```python
from build123d import *

# Parameters (mm, degrees)
SKETCH1_R           = 3.175
BOSS_EXTRUDE1_DEPTH = 3.175
SKETCH2_W           = 63.5
SKETCH2_H           = 25.4
SKETCH2_R           = 3.175
BOSS_EXTRUDE2_DEPTH = 3.175
FILLET1_R           = 2.54


with BuildPart() as part:
    # Sketch1 → Boss-Extrude1 (new body)
    with BuildSketch(Plane.XY):
        with BuildLine():
            Line((-41.275, 55.28710968), (-41.275, -22.225))
            Line((-41.275, -22.225), (22.225, -22.225))
            Line((22.225, -22.225), (22.225, -6.35))
            Line((22.225, -6.35), (-26.194658329, 42.069658329))
            ThreePointArc((-26.194658329, 42.069658329), (-32.769591892, 42.42721549), (-29.935488317, 48.370737627))
            ThreePointArc((-29.935488317, 48.370737627), (-28.368460583, 49.237906002), (-27.763159017, 50.923482141))
            ThreePointArc((-27.763159017, 50.923482141), (-32.032478959, 57.847259125), (-40.154061033, 57.393733943))
            ThreePointArc((-40.154061033, 57.393733943), (-40.977321902, 56.480253631), (-41.275, 55.28710968))
        make_face()
        Circle(SKETCH1_R, mode=Mode.SUBTRACT)
        with Locations((-31.75, 0)):
            Circle(SKETCH1_R, mode=Mode.SUBTRACT)
        with Locations((-31.75, 31.75)):
            Circle(SKETCH1_R, mode=Mode.SUBTRACT)
    extrude(amount=BOSS_EXTRUDE1_DEPTH)

    # Sketch2 → Boss-Extrude2 (add)
    with BuildSketch(Plane(origin=(0, -22.225, 0), x_dir=(1, 0, 0), z_dir=(0, 1, 0))):
        with Locations((-9.525, -15.875)):
            Rectangle(SKETCH2_W, SKETCH2_H)
        with Locations((-9.525, -15.875)):
            Circle(SKETCH2_R, mode=Mode.SUBTRACT)
        with Locations((-31.75, -19.05)):
            Circle(SKETCH2_R, mode=Mode.SUBTRACT)
        with Locations((12.7, -19.05)):
            Circle(SKETCH2_R, mode=Mode.SUBTRACT)
    extrude(amount=BOSS_EXTRUDE2_DEPTH)

    # Fillet1
    fillet1_edges = [part.edges().sort_by_distance(p)[0] for p in [
        (-9.525, -22.225, 0),
    ]]
    fillet(fillet1_edges, radius=FILLET1_R)


solid = part.part
```
The listing builds one solid part. Answer for the finished solid, in the listing's coordinates (mm). A direction names the side the tool comes from. Coordinates: 2 decimals unless noted, no trailing zeros. Loops run counter-clockwise (first coordinate to the right, second up) from the corner with the lowest first, then second, coordinate; pieces in that order, holes last. Notation, with made-up numbers: (-5.5, 1) -> (18.5, 1) arc R21 cw to (18.5, 5) -> close; hole circle Ø9 at (74, 36.5). An arc over 180 degrees is marked (long way). Return JSON: item names as keys, results as strings. Group by question number.
(1) A cutting plane is placed at B-B on x = 12.7. Write down the section's boundary in (y, z) (3 decimals).
(2) Find the intervals of material crossed by probe 1 along Y at (x, z) = (-31.75, 2.2) (3 decimals); probe 2 along Y at (x, z) = (-3, 10.75) (3 decimals); probe 3 along Z at (x, y) = (-15, 0) (3 decimals), in increasing order. Write a range as from..to.
(3) A cutting plane is placed at A-A on y = 0. Write down the section's boundary in (x, z) (3 decimals), and give its area (3 significant figures).
(4) A cutting plane is placed at C-C on z = 17.25. Write down the section's boundary in (x, y) (3 decimals).
(5) A cutting plane is placed at D-D on x = -31.75. Write down the section's boundary in (y, z) (3 decimals).
(6) Determine the mould class of faces 4 (the cylindrical face through (9.53, -20.66, 18.91)), 5 (the flat face through (-10, -21, 28.575)), 6 (the cylindrical face through (-32.71, 42.33, 1.57)) for opening direction Z: released by +Z, released by -Z, zero draft, split by the parting line, or undercut.
(7) Which of the six approach directions +Z, -Z, +X, -X, +Y, -Y give full straight-line access (tool end or side, diameter ignored) to faces 1 (the flat face through (-17, 12, 3.175)), 2 (the cylindrical face through (-31.927, 57.791, 1.565)), 3 (the cylindrical face through (-28.4, 49.2, 1.6))?
(8) Given pin 1 Ø5 at (x, z) = (-31.75, 19.05) entering from -Y; pin 2 Ø9 at (x, y) = (-29.36, 44.45) entering from -Z; pin 3 Ø10 at (x, z) = (12.7, 19.05) entering from +Y; pin 4 Ø10 at (x, y) = (-33.5, -14) entering from +Z (3 decimals), each flat-ended and moving along its own axis, determine where each tip first touches the part or whether it passes through.
The answers:
{
 "1": {"outline": "(-22.225, 2.54) arc R2.54 ccw to (-19.685, 0) -> (3.175, 0) -> (3.175, 3.175) -> (-19.05, 3.175) -> (-19.05, 15.875) -> (-22.225, 15.875) -> close; (-22.225, 22.225) -> (-19.05, 22.225) -> (-19.05, 28.575) -> (-22.225, 28.575) -> close"},
 "2": {"probe 1": "y = -22.202..-3.175, 3.175..28.575, 34.925..41.288, 47.612..57.692", "probe 2": "y = -22.225..-19.05", "probe 3": "z = 0..3.175"},
 "3": {"outline": "(-41.275, 0) -> (-34.925, 0) -> (-34.925, 3.175) -> (-41.275, 3.175) -> close; (-28.575, 0) -> (-3.175, 0) -> (-3.175, 3.175) -> (-28.575, 3.175) -> close; (3.175, 0) -> (15.875, 0) -> (15.875, 3.175) -> (3.175, 3.175) -> close", "area": "141 mm^2"},
 "4": {"outline": "(-41.275, -22.225) -> (-34.365, -22.225) -> (-34.365, -19.05) -> (-41.275, -19.05) -> close; (-29.135, -22.225) -> (-12.387, -22.225) -> (-12.387, -19.05) -> (-29.135, -19.05) -> close; (-6.663, -22.225) -> (10.085, -22.225) -> (10.085, -19.05) -> (-6.663, -19.05) -> close; (15.315, -22.225) -> (22.225, -22.225) -> (22.225, -19.05) -> (15.315, -19.05) -> close"},
 "5": {"outline": "(-22.225, 2.54) arc R2.54 ccw to (-19.685, 0) -> (-3.175, 0) -> (-3.175, 3.175) -> (-19.05, 3.175) -> (-19.05, 15.875) -> (-22.225, 15.875) -> close; (-22.225, 22.225) -> (-19.05, 22.225) -> (-19.05, 28.575) -> (-22.225, 28.575) -> close; (3.175, 0) -> (28.575, 0) -> (28.575, 3.175) -> (3.175, 3.175) -> close; (34.925, 0) -> (41.288, 0) -> (41.288, 3.175) -> (34.925, 3.175) -> close; (47.612, 0) -> (57.692, 0) -> (57.692, 3.175) -> (47.612, 3.175) -> close"},
 "6": {"face 4": "undercut", "face 5": "released by +Z", "face 6": "zero draft"},
 "7": {"face 1": "+Z, +X, -X, +Y", "face 2": "+Z, -Z, +Y", "face 3": "+Z, -Z, +X"},
 "8": {"pin 1": "passes through", "pin 2": "stops at z = 0", "pin 3": "stops at y = -19.05", "pin 4": "stops at z = 3.175"}
}
